Design review of the part built by this model. Coordinates are the model's own, in mm. A direction names the side the tool comes from. Round coordinates to 2 decimals unless told otherwise and drop trailing zeros. Order: outer loops, then holes, each group sorted by start corner. A loop starts at its lowest first (then second) coordinate and runs counter-clockwise, first axis right, second up.
from build123d import *

# Parameters (mm, degrees)
SKETCH_1_W                       = 30
SKETCH_1_H                       = 30
EXTRUDE_1_DEPTH                  = 3
EXTRUDE_2_DEPTH                  = 1.5
FILLET_2_R                       = 10
SKETCH_4_R                       = 51
CUT_EXTRUDE_1_DEPTH              = 80
SKETCH_5_R                       = 1.6
CUT_EXTRUDE_3_DEPTH              = 10
SHEET_EXTRUDE_2_1_DEPTH          = 35
THICKEN_2_T2                     = 3
PATTERN_CIRCULAR_8_COUNT         = 4
FILLET_2_OF_PATTERN_CIRCULAR_8_R = 10
SKETCH_6_R                       = 51
CUT_EXTRUDE_4_DEPTH              = 35


with BuildPart() as part:
    # 草图1 → 凸台-拉伸1 (new body)
    with BuildSketch(Plane(origin=(0, 0, 0), x_dir=(1, 0, 0), z_dir=(0, 1, 0))):
        Rectangle(SKETCH_1_W, SKETCH_1_H)
    extrude_1 = extrude(amount=EXTRUDE_1_DEPTH)

    # 草图3 → 凸台-拉伸2 (add, symmetric)
    with BuildSketch(Plane.XY):
        Polygon((-13, 3), (4.320508076, 33), (50, 33), (50, 3), align=None)
    extrude_2 = extrude(amount=EXTRUDE_2_DEPTH, both=True)

    # 圆角2
    fillet_2_edges = [part.edges().sort_by_distance(p)[0] for p in [
        (-15, 1.5, 15),
        (-15, 1.5, -15),
    ]]
    fillet(fillet_2_edges, radius=FILLET_2_R)

    # 草图4 → 切除-拉伸1 (cut)
    with BuildSketch(Plane(origin=(0, 0, 0), x_dir=(1, 0, 0), z_dir=(0, 1, 0))):
        with Locations((52, 0)):
            Circle(SKETCH_4_R)
    extrude(amount=CUT_EXTRUDE_1_DEPTH, mode=Mode.SUBTRACT)

    # 草图5 → 切除-拉伸3 (cut)
    with BuildSketch(Plane(origin=(0, 0, 0), x_dir=(1, 0, 0), z_dir=(0, 1, 0))):
        with Locations(Location((-8, 8, 0), (0, 0, 90))):
            Circle(SKETCH_5_R)
        with Locations(Location((-8, -8, 0), (0, 0, 90))):
            Circle(SKETCH_5_R)
    cut_extrude_3 = extrude(amount=CUT_EXTRUDE_3_DEPTH, mode=Mode.SUBTRACT)

    # Sheet 凸台-拉伸2: a surface, the sketch's curves swept straight by 35 mm
    with BuildLine(Plane(origin=(0, 0, 0), x_dir=(1, 0, 0), z_dir=(0, 1, 0)), mode=Mode.PRIVATE) as sheet_extrude_2_1_path:
        CenterArc((52, 0), 51, 0, 360)
    sheet_extrude_2_1 = Shell.extrude(sheet_extrude_2_1_path.wire(), (0 * SHEET_EXTRUDE_2_1_DEPTH, 1 * SHEET_EXTRUDE_2_1_DEPTH, 0 * SHEET_EXTRUDE_2_1_DEPTH))
    add(Solid.thicken(sheet_extrude_2_1, -THICKEN_2_T2))

    # 阵列(圆周)8: 凸台-拉伸1, 凸台-拉伸2, 切除-拉伸3 ×4 about axis
    pattern_circular_8_axis = Axis((52, 0, 0), (0, 1, 0))
    add([extrude_1.rotate(pattern_circular_8_axis, i * 360 / PATTERN_CIRCULAR_8_COUNT) for i in range(1, PATTERN_CIRCULAR_8_COUNT)])
    add([extrude_2.rotate(pattern_circular_8_axis, i * 360 / PATTERN_CIRCULAR_8_COUNT) for i in range(1, PATTERN_CIRCULAR_8_COUNT)])
    add([cut_extrude_3.rotate(pattern_circular_8_axis, i * 360 / PATTERN_CIRCULAR_8_COUNT) for i in range(1, PATTERN_CIRCULAR_8_COUNT)], mode=Mode.SUBTRACT)

    # 圆角2 of 阵列(圆周)8
    fillet_2_of_pattern_circular_8_edges = [part.edges().sort_by_distance(p)[0] for p in [
        (67, 1.5, 67),
        (37, 1.5, 67),
        (119, 1.5, -15),
        (119, 1.5, 15),
        (37, 1.5, -67),
        (67, 1.5, -67),
    ]]
    fillet(fillet_2_of_pattern_circular_8_edges, radius=FILLET_2_OF_PATTERN_CIRCULAR_8_R)

    # 草图6 → 切除-拉伸4 (cut)
    with BuildSketch(Plane(origin=(0, 0, 0), x_dir=(1, 0, 0), z_dir=(0, 1, 0))):
        with Locations(Location((52, 0, 0), (0, 0, 270))):
            Circle(SKETCH_6_R)
    extrude(amount=CUT_EXTRUDE_4_DEPTH, mode=Mode.SUBTRACT)


solid = part.part
1) Take a section at B-B on x = 95. Give the boundary of the cut face in (y, z), plus the area to 3 significant figures.
Results:
outline: (0, -32.66) - (35, -32.66) - (35, -27.42) - (0, -27.42) - close; (0, 27.42) - (35, 27.42) - (35, 32.66) - (0, 32.66) - close
area: 367 mm2
2) The part is to be moulded in two halves that separate along Z. For faces 1 (the face through (-12.15, 1.52, 11.99)), 2 (the face through (-8, 3, 3)), 3 (the face through (-2, 1, -15)), 4 (the face through (-7.03, 1.48, -6.73)), say which applies: released by +Z, released by -Z, zero draft, split by the parting line, or undercut.
Results:
face 1: released by +Z
face 2: zero draft
face 3: released by -Z
face 4: undercut
3) To check wall thickness, follow line 1 along Z through (x, y) = (44, 1); line 2 along Z through (x, y) = (-8, 2); line 3 along X through (y, z) = (1.75, 8). State the ranges of each line that lie inside material, in increasing order.
Results:
line 1: z = -66.54 to -61.6, -58.4 to -50.37, 50.37 to 58.4, 61.6 to 66.54
line 2: z = -14.54 to -9.6, -6.4 to 6.4, 9.6 to 14.54
line 3: x = -14.54 to -9.6, -6.4 to 1.63, 102.37 to 110.4, 113.6 to 118.54
4) For faces 5 (the face through (106, 1, -15)), 6 (the face through (112, 3, -3)), 7 (the face through (115.99, 1.52, 12.15)), list the 3-axis set-ups (+Z, -Z, +X, -X, +Y, -Y) from which the entire face can be reached by the end or side of a thin tool; tool diameter is ignored.
Results:
face 5: -Z, +X, +Y, -Y
face 6: +X, +Y
face 7: +Z, +X, +Y, -Y
5) Clearance check with flat-ended pins moving along their axes: P1, Ø0.9, axis at x = 105.5, y = 1, coming from the +Z side; P2, Ø2.5, axis at y = 1, z = -54.5, coming from the +X side; P3, Ø4.5, axis at x = 48, z = -57, coming from the +Y side; P4, Ø3, axis at x = -8, z = -8, coming from the +Y side. State where each tip first meets the part, or that it passes through.
Results:
P1: stops at z = 15
P2: stops at x = 67
P3: stops at y = 3
P4: passes through
6) Take a section at A-A on z = -27. Give the boundary of the cut face in (x, y), plus the area to 3 significant figures.
Results:
outline: (5.23, 0) - (8.73, 0) - (8.73, 35) - (5.23, 35) - close; (95.27, 0) - (98.77, 0) - (98.77, 35) - (95.27, 35) - close
area: 245 mm2
7) Take a section at C-C on y = 6. Give the boundary of the cut face in (x, z).
Results:
outline: (-11.27, -1.5) - (-1.98, -1.5) arc R54 ccw to (50.5, -53.98) - (50.5, -63.27) - (53.5, -63.27) - (53.5, -53.98) arc R54 ccw to (105.98, -1.5) - (115.27, -1.5) - (115.27, 1.5) - (105.98, 1.5) arc R54 ccw to (53.5, 53.98) - (53.5, 63.27) - (50.5, 63.27) - (50.5, 53.98) arc R54 ccw to (-1.98, 1.5) - (-11.27, 1.5) - close; hole circle Ø102 at (52, 0)
